Part model, mm, in its own coordinate system. A direction names the side the tool comes from. Give positions to 0.01 mm unless a question says otherwise; leave off trailing zeros. Write each loop counter-clockwise with the first axis right and the second up, starting at its lowest first coordinate (ties: lowest second). Pieces come first, ordered by that corner, then holes. Notation, with made-up numbers: (44, 30.25) - (91, 30.25) arc R16 cw to (91, 41.25) - close; hole circle Ø5 at (15, 49). An arc over 180 degrees is marked (long way). Answer in a Markdown table with one row per item. Add a question column.
1. Probe line 1 along X through (y, z) = (15.75, 0); line 2 along Y through (x, z) = (-5.5, 10); line 3 along Y through (x, z) = (28, -44.5). List the from-to ranges inside material, lowest first.
2. Band-saw the part on B-B on z = 0. Write the cut outline in (x, y).
3. Band-saw the part on D-D on x = 26.5. Write the cut outline in (y, z), plus the area to 3 significant figures.
4. Which spindle directions (+Z, -Z, +X, -X, +Y, -Y) get a long thin tool onto all of the face, cutting with end or side? Do faces 5 (the cylindrical face through (-1.774, 18.961, 50.705)), 6 (the cylindrical face through (-61.99, 6.26, -13.77)). Say none if no direction does.
5. Band-saw the part on C-C on y = 21.25. State how many separate pieces and enclosed holes the cut face has, plus the area to 3 significant figures.
6. Drop flat-ended pins along their axis: pin 1 Ø5 at (y, z) = (18.5, 3) entering from -X; pin 2 Ø1.5 at (x, y) = (17, 8) entering from -Z; pin 3 Ø5 at (x, y) = (5, 18.5) entering from +Z. Give the stop position or say it passes through.
7. Band-saw the part on A-A on x = 0. Write the cut outline in (y, z) (1 decimal), plus the area to 3 significant figures.
8. Pull direction X, two halves, no side cores. Call faces 1 (the cylindrical face through (0.95, 20.25, -54.12)), 2 (the cylindrical face through (1.926, 14.472, 6.117)), 3 (the cylindrical face through (-0.494, 19.139, -25.403)), 4 (the flat face through (1, 25.4, 15)): released by +X, released by -X, zero draft, split by the parting line, or undercut.
```python
from build123d import *

# Parameters (mm, degrees)
SKETCH1_R           = 63.5
SKETCH1_R_2         = 6.4135
BOSS_EXTRUDE1_DEPTH = 12.7
SKETCH2_R           = 50.7365
SKETCH2_R_2         = 6.4135
BOSS_EXTRUDE2_DEPTH = 12.7
SKETCH3_R           = 38.1
CUT_EXTRUDE2_DEPTH  = 12.7
SKETCH4_R           = 3.175
BOSS_EXTRUDE3_DEPTH = 12.7
FILLET1_R           = 2.54
FILLET2_R           = 5.08
FILLET3_R           = 1.27


with BuildPart() as part:
    # Sketch1 → Boss-Extrude1 (new body)
    with BuildSketch(Plane(origin=(0, 0, 0), x_dir=(1, 0, 0), z_dir=(0, 1, 0))):
        with Locations(Location((0, 0, 0), (0, 0, 270))):
            Circle(SKETCH1_R)
        with Locations(Location((0, 0, 0), (0, 0, 270))):
            Circle(SKETCH1_R_2, mode=Mode.SUBTRACT)
    extrude(amount=BOSS_EXTRUDE1_DEPTH)

    # Sketch2 → Boss-Extrude2 (add)
    with BuildSketch(Plane(origin=(0, 12.7, 0), x_dir=(1, 0, 0), z_dir=(0, 1, 0))):
        with Locations(Location((0, 0, 0), (0, 0, 270))):
            Circle(SKETCH2_R)
        with Locations(Location((0, 0, 0), (0, 0, 270))):
            Circle(SKETCH2_R_2, mode=Mode.SUBTRACT)
    extrude(amount=BOSS_EXTRUDE2_DEPTH)

    # Sketch3 → Cut-Extrude2 (cut)
    with BuildSketch(Plane(origin=(0, 25.4, 0), x_dir=(1, 0, 0), z_dir=(0, 1, 0))):
        with Locations((0, 63.5)):
            Circle(SKETCH3_R)
    extrude(amount=-CUT_EXTRUDE2_DEPTH, mode=Mode.SUBTRACT)

    # Sketch4 → Boss-Extrude3 (add)
    with BuildSketch(Plane(origin=(0, 12.7, 0), x_dir=(1, 0, 0), z_dir=(0, 1, 0))):
        with Locations(Location((0, 57.15, 0), (0, 0, 270))):
            Circle(SKETCH4_R)
    extrude(amount=BOSS_EXTRUDE3_DEPTH)

    # Fillet1
    fillet1_edges = [part.edges().sort_by_distance(p)[0] for p in [
        (0, 12.7, -60.325),
    ]]
    fillet(fillet1_edges, radius=FILLET1_R)

    # Fillet2
    fillet2_edges = [part.edges().sort_by_distance(p)[0] for p in [
        (0, 0, -6.4135),
    ]]
    fillet(fillet2_edges, radius=FILLET2_R)

    # Fillet3
    fillet3_edges = [part.edges().sort_by_distance(p)[0] for p in [
        (0, 25.4, -6.4135),
    ]]
    fillet(fillet3_edges, radius=FILLET3_R)


solid = part.part
```
Values:
| question | item | result |
|---|---|---|
| 1 | line 1 | x = -50.74 to -6.41, 6.41 to 50.74 |
| 1 | line 2 | y = 0 to 25.4 |
| 1 | line 3 | y = 0 to 12.7 |
| 2 | outline | (-63.5, 0) - (-11.49, 0) arc R5.08 ccw to (-6.41, 5.08) - (-6.41, 24.13) arc R1.27 ccw to (-7.68, 25.4) - (-50.74, 25.4) - (-50.74, 12.7) - (-63.5, 12.7) - close; (6.41, 5.08) arc R5.08 ccw to (11.49, 0) - (63.5, 0) - (63.5, 12.7) - (50.74, 12.7) - (50.74, 25.4) - (7.68, 25.4) arc R1.27 ccw to (6.41, 24.13) - close |
| 3 | outline | (0, -57.71) - (12.7, -57.71) - (12.7, -36.13) - (25.4, -36.13) - (25.4, 43.27) - (12.7, 43.27) - (12.7, 57.71) - (0, 57.71) - close |
| 3 | area | 2,470 mm² |
| 4 | face 5 | +Y |
| 4 | face 6 | +Y, -Y |
| 5 | separate pieces | 2 |
| 5 | enclosed holes | 1 |
| 5 | area | 6,920 mm² |
| 6 | pin 1 | stops at x = -50.73 |
| 6 | pin 2 | stops at z = -61.39 |
| 6 | pin 3 | stops at z = 50.67 |
| 7 | outline | (0, -63.5) - (12.7, -63.5) - (12.7, -62.9) arc R2.5 cw to (15.2, -60.3) - (25.4, -60.3) - (25.4, -54) - (15.2, -54) arc R2.5 cw to (12.7, -51.4) - (12.7, -25.4) - (25.4, -25.4) - (25.4, -7.7) arc R1.3 ccw to (24.1, -6.4) - (5.1, -6.4) arc R5.1 ccw to (0, -11.5) - close; (0, 11.5) arc R5.1 ccw to (5.1, 6.4) - (24.1, 6.4) arc R1.3 ccw to (25.4, 7.7) - (25.4, 50.7) - (12.7, 50.7) - (12.7, 63.5) - (0, 63.5) - close |
| 7 | area | 2,330 mm² |
| 8 | face 1 | split by the parting line |
| 8 | face 2 | undercut |
| 8 | face 3 | undercut |
| 8 | face 4 | zero draft |
